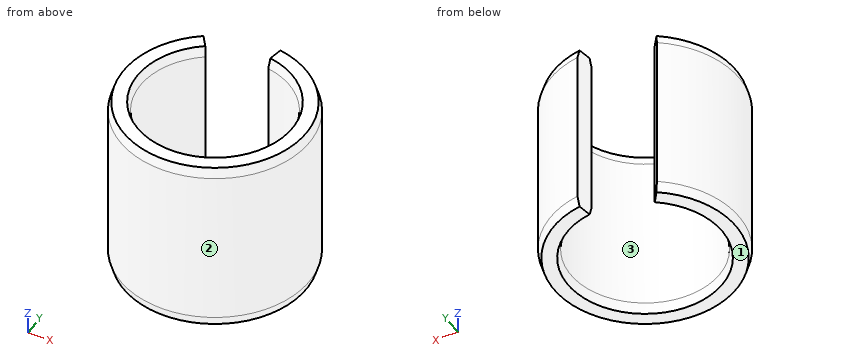
```python
from build123d import *

# Parameters (mm, degrees)
F1_DEPTH   = 18
F2_SIZE2   = 1
F2_SIZE    = 0.3
F2_2_SIZE2 = 1
F2_2_SIZE  = 0.3


# Not quite as in the source:
# - a feature names something its author has since deleted; it is built from what else it names


with BuildPart() as f1:
    # F0 (on Top) → F1 (new body)
    with BuildSketch(Plane.XY):
        with BuildLine():
            ThreePointArc((1.2044566856, 7.40527886), (1.7499452086, -7.2956536834), (-4.4326164701, 6.0531629856))
            Line((-4.4326164701, 6.0531629856), (-5.6190034408, 7.6732881976))
            ThreePointArc((-5.6190034408, 7.6732881976), (2.2183169274, -9.2483307381), (1.5268287492, 9.3872970232))
            Line((1.5268287492, 9.3872970232), (1.2044566856, 7.40527886))
        make_face()
    extrude(amount=F1_DEPTH)

    # F2
    f2_edges = [f1.edges().sort_by_distance(p)[0] for p in [
        (2.218317, -9.248331, 18),
        (1.749945, -7.295654, 18),
    ]]
    f2_side = f1.faces().sort_by_distance((1.630296, 8.353243, 18))[0]
    chamfer(f2_edges, length=F2_SIZE, length2=F2_SIZE2, reference=f2_side)

    # F2#2
    f2_2_edges = [f1.edges().sort_by_distance(p)[0] for p in [
        (2.218317, -9.248331, 0),
        (1.749945, -7.295654, 0),
    ]]
    f2_2_side = f1.faces().sort_by_distance((1.630296, 8.353243, 0))[0]
    chamfer(f2_2_edges, length=F2_2_SIZE, length2=F2_2_SIZE2, reference=f2_2_side)


solid = f1.part
```
Geometry: final body of the model. Coordinates: model frame, mm. Face numbers are marked on the shaded views. Coordinates: 2 decimals unless noted, no trailing zeros. Order: outer loops, then holes, each group sorted by start corner. A loop starts at its lowest first (then second) coordinate and runs counter-clockwise, first axis right, second up. Notation, with made-up numbers: (-3, 18.25) -> (7, 18.25) arc R12 ccw to (7, 36.25) -> close; hole circle Ø1 at (5, 88). An arc over 180 degrees is marked (long way). Use CSV: the item, a comma, the result in double quotes.
1) Line query: line 1 (X direction, y = 0, z = 13); line 2 (Y direction, x = 0, z = 17); line 3 (Y direction, x = 6.5, z = 10.25). Output: solid intervals per line, ascending.
Findings:
line 1,"x = -9.51 to -7.5, 7.5 to 9.51"
line 2,"y = -9.51 to -7.5"
line 3,"y = -6.94 to -3.75, 3.75 to 6.94"
2) Pin query (flat end, axial travel): pin 1 Ø2 at (x, z) = (7.5, 14.5) entering from -Y; pin 2 Ø2 at (x, z) = (-2, 15.5) entering from +Y; pin 3 Ø1.5 at (y, z) = (1, 6.5) entering from -X. Return the tip coordinate at first contact, or that it passes through.
Findings:
pin 1,"stops at y = -6.94"
pin 2,"stops at y = -6.88"
pin 3,"stops at x = -9.51"
3) Section C-C on z = 2.5. Output: boundary loops of the cut face in (x, y), then the cut area to 3 significant figures.
Findings:
outline,"(-5.62, 7.67) arc R9.51 ccw (long way) to (1.53, 9.39) -> (1.2, 7.41) arc R7.5 cw (long way) to (-4.43, 6.05) -> close"
area,"93.8 mm^2"
4) Section B-B on x = 0. Output: boundary loops of the cut face in (y, z), then the cut area to 3 significant figures.
Findings:
outline,"(-9.51, 1) -> (-9.21, 0) -> (-7.8, 0) -> (-7.5, 1) -> (-7.5, 17) -> (-7.8, 18) -> (-9.21, 18) -> (-9.51, 17) -> close"
area,"35.5 mm^2"
5) Section A-A on y = 0. Output: boundary loops of the cut face in (x, z), then the cut area to 3 significant figures.
Findings:
outline,"(-9.51, 1) -> (-9.21, 0) -> (-7.8, 0) -> (-7.5, 1) -> (-7.5, 17) -> (-7.8, 18) -> (-9.21, 18) -> (-9.51, 17) -> close; (7.5, 1) -> (7.8, 0) -> (9.21, 0) -> (9.51, 1) -> (9.51, 17) -> (9.21, 18) -> (7.8, 18) -> (7.5, 17) -> close"
area,"71.1 mm^2"
6) Mould query, pull axis Y, two halves, no side actions, for the marked faces 1, 2 and 3. Classes: +Y half, -Y half, draft (parallel to the pull), parting line (faces both ways), or undercut.
Findings:
face 1,"draft"
face 2,"parting line"
face 3,"undercut"
